Part model, mm, in its own coordinate system. A direction names the side the tool comes from. Round coordinates to 2 decimals unless told otherwise and drop trailing zeros. Write each loop counter-clockwise with the first axis right and the second up, starting at its lowest first coordinate (ties: lowest second). Pieces come first, ordered by that corner, then holes. Notation, with made-up numbers: M 70,28 L 101,28 A34 ccw 101,63 Z; hole C 88.5,5 d8. An arc over 180 degrees is marked long. Use a Markdown table: item, result. Add a question column.
1) Slice it at D-D on x = -26.5. Write the cut outline in (y, z), plus the area to 3 significant figures.
2) Slice it at C-C on z = 0. Give the number of separate pieces and of enclosed holes in the cut face, plus the area to 3 significant figures.
3) Slice it at A-A on y = 62. Write the cut outline in (x, z).
4) Two-plate mould, pull along Z, no slides. Class faces 1 (the face through (35, 58, 0)), 2 (the face through (-39.86, 23.12, -15.63)): released by +Z, released by -Z, zero draft, split by the parting line, or undercut.
5) Which spindle directions (+Z, -Z, +X, -X, +Y, -Y) get a long thin tool onto all of the face, cutting with end or side? Do faces 3 (the face through (0, 6, 0)), 4 (the face through (39, 35, 4)), 5 (the face through (35.99, 23.65, 10.84)), 6 (the face through (0, 9, -1)), 7 (the face through (6, 7, 0)). Say none if no direction does.
6) Wall check: probe 1 along X at (y, z) = (2.1, 0); probe 2 along Y at (x, z) = (22.5, -38); probe 3 along Y at (x, z) = (-44, -4.5). Give the ranges that are in metal, low to high.
7) Drop flat-ended pins along their axis: P1, Ø2.5, axis at x = -3.75, z = -6.5, coming from the -Y side; P2, Ø8, axis at x = -28, z = -35.5, coming from the +Y side; P3, Ø13.5, axis at y = 45.5, z = -5, coming from the -X side; P4, Ø23.5, axis at y = 36, z = -11.5, coming from the -X side. Give the stop position or say it passes through.
8) Slice it at B-B on x = -3.75. Write the cut outline in (y, z), plus the area to 3 significant figures.
```python
from build123d import *

# Parameters (mm, degrees)
CROQUIS1_R              = 47.5
CROQUIS1_R_2            = 10
SALIENTE_EXTRUIR1_DEPTH = 6
CROQUIS2_R              = 47.5
CROQUIS2_R_2            = 1.5
SALIENTE_EXTRUIR2_DEPTH = 3
CROQUIS3_R              = 45
CROQUIS3_R_2            = 32.5
CORTAR_EXTRUIR1_DEPTH   = 3
CROQUIS4_R              = 13.5
CORTAR_EXTRUIR2_DEPTH   = 4
SALIENTE_EXTRUIR4_DEPTH = 70
REDONDEO1_R             = 10
CROQUIS6_R              = 13.5
CORTAR_EXTRUIR3_DEPTH   = 4
CROQUIS7_R              = 10
CORTAR_EXTRUIR4_DEPTH   = 124.707316002
CROQUIS8_R              = 23.5
CROQUIS8_R_2            = 15
CORTAR_EXTRUIR5_DEPTH   = 2
CROQUIS10_R             = 16
CORTAR_EXTRUIR6_DEPTH   = 124.707316002
CROQUIS12_R             = 1.52
CORTAR_EXTRUIR8_DEPTH   = 124.707316002


with BuildPart() as part:
    # Croquis1 → Saliente-Extruir1 (new body)
    with BuildSketch(Plane(origin=(0, 0, 0), x_dir=(1, 0, 0), z_dir=(0, 1, 0))):
        with Locations(Location((0, 0, 0), (0, 0, 270))):
            Circle(CROQUIS1_R)
        with Locations(Location((0, 0, 0), (0, 0, 270))):
            Circle(CROQUIS1_R_2, mode=Mode.SUBTRACT)
    extrude(amount=SALIENTE_EXTRUIR1_DEPTH)

    # Croquis2 → Saliente-Extruir2 (add)
    with BuildSketch(Plane(origin=(0, 6, 0), x_dir=(1, 0, 0), z_dir=(0, 1, 0))):
        with Locations(Location((0, 0, 0), (0, 0, 270))):
            Circle(CROQUIS2_R)
        with Locations(Location((7.5, 0, 0), (0, 0, 270))):
            Circle(CROQUIS2_R_2, mode=Mode.SUBTRACT)
        with Locations(Location((3.75, -6.495190528, 0), (0, 0, 270))):
            Circle(CROQUIS2_R_2, mode=Mode.SUBTRACT)
        with Locations(Location((-3.75, -6.495190528, 0), (0, 0, 270))):
            Circle(CROQUIS2_R_2, mode=Mode.SUBTRACT)
        with Locations(Location((-7.5, 0, 0), (0, 0, 270))):
            Circle(CROQUIS2_R_2, mode=Mode.SUBTRACT)
        with Locations(Location((-3.75, 6.495190528, 0), (0, 0, 270))):
            Circle(CROQUIS2_R_2, mode=Mode.SUBTRACT)
        with Locations(Location((3.75, 6.495190528, 0), (0, 0, 270))):
            Circle(CROQUIS2_R_2, mode=Mode.SUBTRACT)
    extrude(amount=SALIENTE_EXTRUIR2_DEPTH)

    # Croquis3 → Cortar-Extruir1 (cut)
    with BuildSketch(Plane.XZ):
        with Locations(Location((0, 0, 0), (0, 0, 270))):
            Circle(CROQUIS3_R)
        with Locations(Location((0, 0, 0), (0, 0, 270))):
            Circle(CROQUIS3_R_2, mode=Mode.SUBTRACT)
    extrude(amount=-CORTAR_EXTRUIR1_DEPTH, mode=Mode.SUBTRACT)

    # Croquis4 → Cortar-Extruir2 (cut)
    with BuildSketch(Plane.XZ):
        with Locations(Location((0, 0, 0), (0, 0, 270))):
            Circle(CROQUIS4_R)
    extrude(amount=-CORTAR_EXTRUIR2_DEPTH, mode=Mode.SUBTRACT)

    # Croquis5 → Saliente-Extruir4 (add)
    with BuildSketch(Plane(origin=(0, 9, 0), x_dir=(1, 0, 0), z_dir=(0, 1, 0))):
        with BuildLine():
            Line((35, 32.113081447), (35, -32.113081447))
            ThreePointArc((35, -32.113081447), (47.5, 0), (35, 32.113081447))
        make_face()
        with BuildLine():
            Line((-35, 32.113081447), (-35, -32.113081447))
            ThreePointArc((-35, -32.113081447), (-47.5, 0), (-35, 32.113081447))
        make_face()
    extrude(amount=SALIENTE_EXTRUIR4_DEPTH)

    # Redondeo1
    redondeo1_edges = [part.edges().sort_by_distance(p)[0] for p in [
        (47.5, 79, 0),
        (-47.5, 79, 0),
    ]]
    fillet(redondeo1_edges, radius=REDONDEO1_R)

    # Croquis6 → Cortar-Extruir3 (cut)
    with BuildSketch(Plane.ZY.offset(-35)):
        with Locations((0, 44)):
            Circle(CROQUIS6_R)
    extrude(amount=-CORTAR_EXTRUIR3_DEPTH, mode=Mode.SUBTRACT)

    # Croquis7 → Cortar-Extruir4 (cut, through all)
    with BuildSketch(Plane.ZY.offset(-35)):
        with Locations((0, 44.554429855)):
            Circle(CROQUIS7_R)
    extrude(amount=-CORTAR_EXTRUIR4_DEPTH, mode=Mode.SUBTRACT)

    # Croquis8 → Cortar-Extruir5 (cut)
    with BuildSketch(Plane.ZY.offset(-35)):
        with Locations((0, 44.5)):
            Circle(CROQUIS8_R)
        with Locations((0, 44.5)):
            Circle(CROQUIS8_R_2, mode=Mode.SUBTRACT)
    extrude(amount=-CORTAR_EXTRUIR5_DEPTH, mode=Mode.SUBTRACT)

    # Croquis10 → Cortar-Extruir6 (cut, through all)
    with BuildSketch(Plane(origin=(-35, 0, 0), x_dir=(0, 0, -1), z_dir=(1, 0, 0))):
        with Locations((0, 44.554429855)):
            Circle(CROQUIS10_R)
    extrude(amount=-CORTAR_EXTRUIR6_DEPTH, mode=Mode.SUBTRACT)

    # Croquis12 → Cortar-Extruir8 (cut, through all)
    with BuildSketch(Plane(origin=(-35, 0, 0), x_dir=(0, 0, -1), z_dir=(1, 0, 0))):
        with Locations((27.5, 44.554429855)):
            Circle(CROQUIS12_R)
        with Locations((17.149432951, 23.052396202)):
            Circle(CROQUIS12_R)
        with Locations((-6.115006895, 17.73849668)):
            Circle(CROQUIS12_R)
        with Locations((-24.774721825, 32.614206013)):
            Circle(CROQUIS12_R)
        with Locations((-24.778565909, 56.477811664)):
            Circle(CROQUIS12_R)
        with Locations((-6.123644473, 71.35953185)):
            Circle(CROQUIS12_R)
        with Locations((17.142506151, 66.053127737)):
            Circle(CROQUIS12_R)
    extrude(amount=-CORTAR_EXTRUIR8_DEPTH, mode=Mode.SUBTRACT)


solid = part.part
```
Entries:
| question | item | result |
|---|---|---|
| 1 | outline | M 0,-39.42 L 9,-39.42 L 9,39.42 L 0,39.42 L 0,36.37 L 3,36.37 L 3,18.81 L 0,18.81 L 0,-18.81 L 3,-18.81 L 3,-36.37 L 0,-36.37 Z |
| 1 | area | 604 mm^2 |
| 2 | separate pieces | 5 |
| 2 | enclosed holes | 0 |
| 2 | area | 1,610 mm^2 |
| 3 | outline | M -35,-32.11 L -35,32.11 A47.5 ccw Z; M 35,-32.11 A47.5 ccw 35,32.11 L 35,15.68 L 37,15.68 L 37,-15.68 L 35,-15.68 Z |
| 4 | face 1 | zero draft |
| 4 | face 2 | undercut |
| 5 | face 3 | -Y |
| 5 | face 4 | -X |
| 5 | face 5 | none |
| 5 | face 6 | +Z, -Z, +Y |
| 5 | face 7 | +Y, -Y |
| 6 | probe 1 | x = -47.5 to -45, -32.5 to -13.5, 13.5 to 32.5, 45 to 47.5 |
| 6 | probe 2 | y = 3 to 9 |
| 6 | probe 3 | y = 3 to 29.2, 59.91 to 76.4 |
| 7 | P1 | passes through |
| 7 | P2 | stops at y = 9 |
| 7 | P3 | stops at x = 39 |
| 7 | P4 | stops at x = -47.45 |
| 8 | outline | M 0,-47.35 L 9,-47.35 L 9,-8 L 6,-8 L 6,-9.27 L 4,-9.27 L 4,-12.97 L 0,-12.97 L 0,-32.28 L 3,-32.28 L 3,-44.84 L 0,-44.84 Z; M 0,12.97 L 4,12.97 L 4,9.27 L 6,9.27 L 6,8 L 9,8 L 9,47.35 L 0,47.35 L 0,44.84 L 3,44.84 L 3,32.28 L 0,32.28 Z; M 6,-5 L 9,-5 L 9,5 L 6,5 Z |
| 8 | area | 618 mm^2 |
